from build123d import *

# Parameters (mm, degrees)
BOSS_EXTRUDE1_DEPTH = 0.5


with BuildPart() as part:
    # Sketch1 → Boss-Extrude1 (new body)
    with BuildSketch(Plane(origin=(0, 0, 0), x_dir=(1, 0, 0), z_dir=(0, 1, 0))):
        Polygon((-30.973296771, 20.942182778), (-30.973296771, 22.692182778), (-27.973296771, 22.692182778), (-27.973296771, 22.192182778), (-27.973296771, 21.442182778), (-27.973296771, 20.942182778), align=None)
        Polygon((-27.973296771, 22.192182778), (-27.973296771, 21.442182778), (-20.473296771, 21.442182778), (-20.473296771, 24.576066254), (-21.857180247, 24.576066254), (-20.973296771, 23.692182778), (-20.973296771, 22.192182778), align=None)
    extrude(amount=BOSS_EXTRUDE1_DEPTH)


solid = part.part
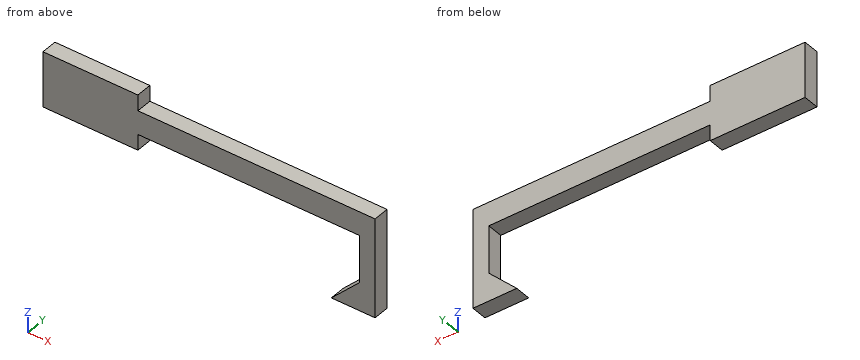
Could you check a few things on this model? Use its own coordinates, in mm. Round coordinates to 2 decimals unless told otherwise and drop trailing zeros. Order: outer loops, then holes, each group sorted by start corner. A loop starts at its lowest first (then second) coordinate and runs counter-clockwise, first axis right, second up.
(1) I'm going to push a flat-ended pin straight in: pin 1 (2 mm diameter, centred on x = -24, z = -22, fed in from -Y). Where does the tip first touch, or does it pass through?
Response values:
pin 1: stops at y = 0
(2) Imagine slicing it at A-A (y = 0.15). Write out the boundary of the cut face in (x, z).
Response values:
outline: (-30.97, -22.69) - (-27.97, -22.69) - (-27.97, -22.19) - (-20.97, -22.19) - (-20.97, -23.69) - (-21.86, -24.58) - (-20.47, -24.58) - (-20.47, -21.44) - (-27.97, -21.44) - (-27.97, -20.94) - (-30.97, -20.94) - close
(3) Imagine slicing it at C-C (x = -28.75). Write out the boundary of the cut face in (y, z).
Response values:
outline: (0, -22.69) - (0.5, -22.69) - (0.5, -20.94) - (0, -20.94) - close
(4) Imagine slicing it at B-B (z = -23.45). Write out the boundary of the cut face in (x, y), plus the area to 3 significant figures.
Response values:
outline: (-20.97, 0) - (-20.47, 0) - (-20.47, 0.5) - (-20.97, 0.5) - close
area: 0.250 mm2
(5) Please list where these lines run through material, in increasing order: line 1 along X through (y, z) = (0.15, -23.35); line 2 along Z through (x, y) = (-24.75, 0.25); line 3 along Z through (x, y) = (-30, 0.3).
Response values:
line 1: x = -20.97 to -20.47
line 2: z = -22.19 to -21.44
line 3: z = -22.69 to -20.94
